Check sheet for the modelled part. Datum: model origin and axes. Units: mm. Face numbers are marked on the shaded views. Coordinates: 2 decimals unless noted, no trailing zeros. Loops run counter-clockwise (first coordinate to the right, second up) from the corner with the lowest first, then second, coordinate; pieces in that order, holes last. Notation, with made-up numbers: M 0.25,15.5 L 21.25,15.5 A18 cw 21.25,20.5 Z; hole C 38.5,5.25 d3. An arc over 180 degrees is marked long. Use CSV: the item, a comma, the result in double quotes. Start each with the question number.
(1) Go/stop test with flat-tipped pins: pin 1 Ø5 at (y, z) = (0, 8) entering from +X; pin 2 Ø4 at (x, z) = (-4, 2) entering from -Y. Record where each tip stops, or that it passes through.
(2) Section check B-B on y = 0. Give the number of separate pieces and of enclosed holes in the cut face, and give its area (3 significant figures).
(3) Section check A-A on x = -0.25. Record the cut outline in (y, z), and give its area (3 significant figures).
(4) Scan lines: line 1 (Z direction, x = 1.25, y = 0); line 2 (Y direction, x = -3, z = -8). Record each from-to range of solid material in increasing order.
(5) Draft check along Y on the marked faces 1, 2 and 3. Enter one of: pulls with the +Y half, pulls with the -Y half, needs draft (parallel to the pull), parting line crosses it, or undercut.
from build123d import *

# Parameters (mm, degrees)
BOSS_EXTRUDE1_DEPTH     = 9
LPATTERN1_COUNT         = 12
LPATTERN1_PITCH         = 1.5
CUT_EXTRUDE1_DEPTH      = 30.538110975
CUT_EXTRUDE1_DEPTH_BACK = 30.538110975
SKETCH5_R               = 2.75


with BuildPart() as part:
    # Sketch2 → Boss-Extrude1 (new, symmetric)
    with BuildSketch(Plane(origin=(0, 0, 0), x_dir=(0, 0, -1), z_dir=(1, 0, 0))):
        with BuildLine():
            Line((16, -6.5), (-16, -6.5))
            ThreePointArc((-16, -6.5), (-22.5, 0), (-16, 6.5))
            Line((-16, 6.5), (16, 6.5))
            ThreePointArc((16, 6.5), (22.5, 0), (16, -6.5))
        make_face()
    extrude(amount=BOSS_EXTRUDE1_DEPTH, both=True)

    # Cut-Sweep1: sweep along a path in Sketch4
    with BuildLine(Plane.ZY.offset(9)) as cut_sweep1_path:
        Line((-16, -6.5), (16, -6.5))
        ThreePointArc((16, -6.5), (22.5, 0), (16, 6.5))
        Line((16, 6.5), (-16, 6.5))
        ThreePointArc((-16, 6.5), (-22.5, 0), (-16, -6.5))
    # Sketch3 → Cut-Sweep1 (sweep, cut)
    with BuildSketch(Plane.XY):
        Polygon((-8.747493318, 6.5), (-8.497493318, 6.066987298), (-8.247493318, 6.5), align=None)
    cut_sweep1 = sweep(path=cut_sweep1_path.line, mode=Mode.SUBTRACT)

    # LPattern1: Cut-Sweep1 ×12
    with Locations(*[(i * LPATTERN1_PITCH, 0, 0) for i in range(1, LPATTERN1_COUNT)]):
        add(cut_sweep1, mode=Mode.SUBTRACT)

    # Sketch5 → Cut-Extrude1 (cut, two sides: drawn at the far end of the back side and taken through both)
    with BuildSketch(Plane(origin=(9, 0, 0), x_dir=(0, 0, -1), z_dir=(1, 0, 0)).offset(-CUT_EXTRUDE1_DEPTH_BACK)):
        with Locations((-8, 0)):
            Circle(SKETCH5_R)
        with Locations((8, 0)):
            Circle(SKETCH5_R)
    extrude(amount=CUT_EXTRUDE1_DEPTH + CUT_EXTRUDE1_DEPTH_BACK, mode=Mode.SUBTRACT)


solid = part.part
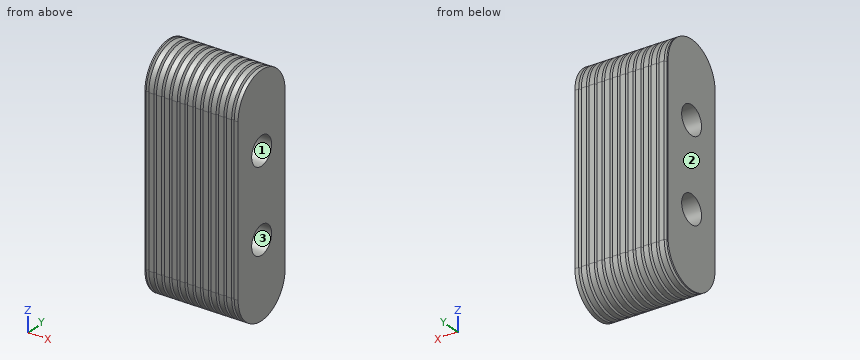
Outcome:
1,pin 1,"passes through"
1,pin 2,"stops at y = -6.5"
2,separate pieces,"3"
2,enclosed holes,"0"
2,area,"609 mm²"
3,outline,"M -6.5,-16 A6.5 ccw 6.5,-16 L 6.5,16 A6.5 ccw -6.5,16 Z; hole C 0,-8 d5.5; hole C 0,8 d5.5"
3,area,"501 mm²"
4,line 1,"z = -22.5 to -10.75, -5.25 to 5.25, 10.75 to 22.5"
4,line 2,"y = -6.5 to -2.75, 2.75 to 6.5"
5,face 1,"undercut"
5,face 2,"needs draft"
5,face 3,"undercut"
